Source: three-view drawing plus pictorial views. Frame: mm from the lowest corner of the part. A direction names the side the tool comes from. Round coordinates to 2 decimals unless told otherwise and drop trailing zeros. Loops run counter-clockwise (first coordinate to the right, second up) from the corner with the lowest first, then second, coordinate; pieces in that order, holes last. Notation, with made-up numbers: (-29.5, -21.75) -> (-17.5, -21.75) arc R22 ccw to (-17.5, -10.75) -> close; hole circle Ø1 at (88.25, 86). An arc over 180 degrees is marked (long way). Put each result on its own line as item: value. Start each with the question number.
1. Cut plane A-A (z = 5.5). Return the cut outline in (x, y) (3 decimals).
2. Cut plane B-B (x = 1.75). Return the cut outline in (y, z), then the cut area to 3 significant figures.
3. Material intervals for L1, parallel to Y at x = 1.75, z = 1; L2, parallel to Y at x = 25, z = 9 (3 decimals); L3, parallel to Z at x = 16.5, y = 7.5, sorted ascending.
4. Contact query for flat-ended pins moving along their axis: pin 1 (5.5 mm diameter, centred on y = 12, z = 6, fed in from -X); pin 2 (5 mm diameter, centred on x = 9.5, y = 12, fed in from +Z). Output: stop coordinate, or through.
5. Cut plane D-D (x = 31.5). Return the cut outline in (y, z) (3 decimals).
6. Set-up query: the marked faces 1, 2 and 3. Return all of +Z, -Z, +X, -X, +Y, -Y with unobstructed straight access to the full face (end or side cutting, diameter ignored); none if empty.
7. Cut plane C-C (y = 1.7). Return the cut outline in (x, z).
8. Draft query along Z for the marked faces 4, 5 and 6. Return one class per face: pulls with the +Z half, pulls with the -Z half, needs draft (parallel to the pull), parting line crosses it, or undercut.
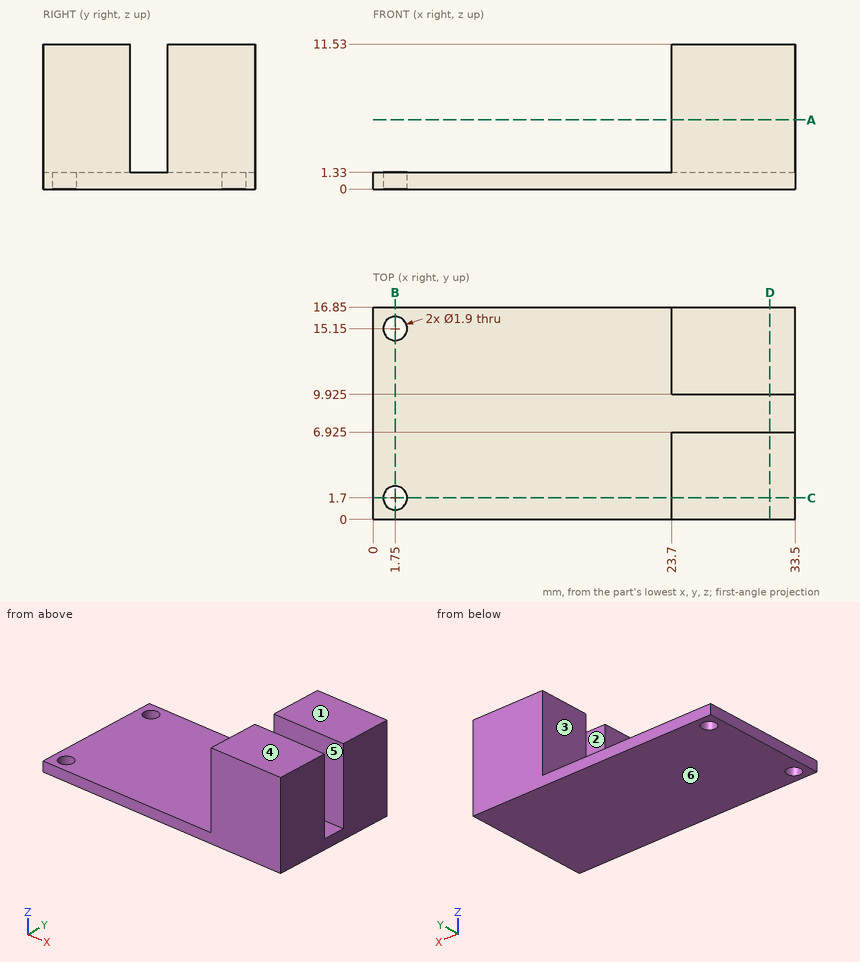
Solution:
1. outline: (23.7, 0) -> (33.5, 0) -> (33.5, 6.925) -> (23.7, 6.925) -> close; (23.7, 9.925) -> (33.5, 9.925) -> (33.5, 16.85) -> (23.7, 16.85) -> close
2. outline: (0, 0) -> (0.75, 0) -> (0.75, 1.33) -> (0, 1.33) -> close; (2.65, 0) -> (14.2, 0) -> (14.2, 1.33) -> (2.65, 1.33) -> close; (16.1, 0) -> (16.85, 0) -> (16.85, 1.33) -> (16.1, 1.33) -> close
2. area: 17.4 mm^2
3. L1: y = 0 to 0.75, 2.65 to 14.2, 16.1 to 16.85
3. L2: y = 0 to 6.925, 9.925 to 16.85
3. L3: z = 0 to 1.33
4. pin 1: stops at x = 23.7
4. pin 2: stops at z = 1.33
5. outline: (0, 0) -> (16.85, 0) -> (16.85, 11.53) -> (9.925, 11.53) -> (9.925, 1.33) -> (6.925, 1.33) -> (6.925, 11.53) -> (0, 11.53) -> close
6. face 1: +Z, +X, -X, +Y, -Y
6. face 2: +Z, +X, -X
6. face 3: +Z, -X, +Y, -Y
7. outline: (0, 0) -> (0.8, 0) -> (0.8, 1.33) -> (0, 1.33) -> close; (2.7, 0) -> (33.5, 0) -> (33.5, 11.53) -> (23.7, 11.53) -> (23.7, 1.33) -> (2.7, 1.33) -> close
8. face 4: pulls with the +Z half
8. face 5: needs draft
8. face 6: pulls with the -Z half
